Design review of the part built by this model. Coordinates are the model's own, in mm. A direction names the side the tool comes from. Coordinates: 2 decimals unless noted, no trailing zeros. Write each loop counter-clockwise with the first axis right and the second up, starting at its lowest first coordinate (ties: lowest second). Pieces come first, ordered by that corner, then holes. Notation, with made-up numbers: (35.25, 45.25) - (61.25, 45.25) arc R17 cw to (61.25, 69.25) - close; hole circle Ø9 at (71.5, 51). An arc over 180 degrees is marked (long way). Answer as a JSON object with one key per item and string values.
```python
from build123d import *

# Parameters (mm, degrees)
SKETCH1_W               = 5
SKETCH1_H               = 5
SKETCH1_R               = 0.95
CENTER_DEPTH            = 1.3
RIGHTSIDE_START         = 1.3
SKETCH1_2_W             = 5
SKETCH1_2_H             = 5
SKETCH1_2_R             = 0.95
RIGHTSIDE_DEPTH         = 1.2
LEFTSIDE_START          = -1.3
SKETCH1_3_W             = 5
SKETCH1_3_H             = 5
SKETCH1_3_R             = 0.95
LEFTSIDE_DEPTH          = 1.2
SKETCH3_W               = 5
SKETCH3_H               = 5
BOSS_EXTRUDE4_DEPTH     = 47.5
CUT_EXTRUDE1_DEPTH      = 5
CIRPATTERN2_COUNT       = 6
CIRPATTERN3_COUNT       = 3
CIRPATTERN4_START       = -44.601270189
CIRPATTERN4_OUTLINE_W   = 5
CIRPATTERN4_OUTLINE_H   = 5
CIRPATTERN4_OUTLINE_R   = 0.95
CIRPATTERN4_DEPTH       = 2.6
CIRPATTERN4_2_OUTLINE_W = 5
CIRPATTERN4_2_OUTLINE_H = 5
CIRPATTERN4_2_OUTLINE_R = 0.95
CIRPATTERN4_2_DEPTH     = 2.6
CIRPATTERN4_START_2     = -1.3
CIRPATTERN4_3_OUTLINE_W = 5
CIRPATTERN4_3_OUTLINE_H = 5
CIRPATTERN4_3_OUTLINE_R = 0.95
CIRPATTERN4_3_DEPTH     = 2.6
SKETCH5_W               = 5
SKETCH5_H               = 2.6
CUT_EXTRUDE2_DEPTH      = 5
INTERSECT1_START        = -46.716333699
INTERSECT1_OUTLINE_W    = 105
INTERSECT1_OUTLINE_H    = 5
INTERSECT1_OUTLINE_R    = 0.95
INTERSECT1_DEPTH        = 49.216333699


# Read off the part's stored shape, not the designer's step: CirPattern4, Intersect1
with BuildPart() as part:
    # Sketch1 → Center (new, symmetric)
    with BuildSketch(Plane(origin=(0, 0, 0), x_dir=(1, 0, 0), z_dir=(0, 1, 0))):
        Rectangle(SKETCH1_W, SKETCH1_H)
        with Locations(Location((0, 0, 0), (0, 0, 270))):
            Circle(SKETCH1_R, mode=Mode.SUBTRACT)
    extrude(amount=CENTER_DEPTH, both=True)

    # Sketch5 → Cut-Extrude2 (cut)
    with BuildSketch(Plane(origin=(2.5, 0, 0), x_dir=(0, 0, -1), z_dir=(1, 0, 0))):
        Rectangle(SKETCH5_W, SKETCH5_H)
    extrude(amount=-CUT_EXTRUDE2_DEPTH, mode=Mode.SUBTRACT)


with BuildPart() as body_2:
    # Sketch1<2> → RightSide (new body)
    with BuildSketch(Plane(origin=(0, 0, 0), x_dir=(1, 0, 0), z_dir=(0, 1, 0)).offset(RIGHTSIDE_START)):
        Rectangle(SKETCH1_2_W, SKETCH1_2_H)
        with Locations(Location((0, 0, 0), (0, 0, 270))):
            Circle(SKETCH1_2_R, mode=Mode.SUBTRACT)
    extrude(amount=RIGHTSIDE_DEPTH)


with BuildPart() as body_3:
    # Sketch1<3> → LeftSide (new body)
    with BuildSketch(Plane(origin=(0, 0, 0), x_dir=(1, 0, 0), z_dir=(0, 1, 0)).offset(LEFTSIDE_START)):
        Rectangle(SKETCH1_3_W, SKETCH1_3_H)
        with Locations(Location((0, 0, 0), (0, 0, 270))):
            Circle(SKETCH1_3_R, mode=Mode.SUBTRACT)
    extrude(amount=-LEFTSIDE_DEPTH)


with BuildPart() as body_4:
    # Sketch3 → Boss-Extrude4 (new body)
    with BuildSketch(Plane.ZY.offset(2.5)):
        Rectangle(SKETCH3_W, SKETCH3_H)
    extrude(amount=BOSS_EXTRUDE4_DEPTH)

    # Sketch4 → Cut-Extrude1 (cut)
    with BuildSketch(Plane.XY.offset(-2.5)):
        Polygon((-50, 0), (-50, -2.5), (-45.669872981, -2.5), align=None)
        Polygon((-50, 2.5), (-50, 0), (-45.669872981, 2.5), align=None)
    extrude(amount=CUT_EXTRUDE1_DEPTH, mode=Mode.SUBTRACT)


with BuildPart() as cirpattern2_1:
    # CirPattern2: pattern copy
    add(body_4.part.rotate(Axis((-50, 0, 0), (0, 0, 1)), 1 * 360 / CIRPATTERN2_COUNT))


with BuildPart() as cirpattern2_2:
    # CirPattern2: pattern copy
    add(body_4.part.rotate(Axis((-50, 0, 0), (0, 0, 1)), 2 * 360 / CIRPATTERN2_COUNT))


with BuildPart() as cirpattern2_3:
    # CirPattern2: pattern copy
    add(body_4.part.rotate(Axis((-50, 0, 0), (0, 0, 1)), 3 * 360 / CIRPATTERN2_COUNT))


with BuildPart() as cirpattern2_4:
    # CirPattern2: pattern copy
    add(body_4.part.rotate(Axis((-50, 0, 0), (0, 0, 1)), 4 * 360 / CIRPATTERN2_COUNT))


with BuildPart() as cirpattern2_5:
    # CirPattern2: pattern copy
    add(body_4.part.rotate(Axis((-50, 0, 0), (0, 0, 1)), 5 * 360 / CIRPATTERN2_COUNT))


with BuildPart() as cirpattern3_1:
    # CirPattern3: pattern copy
    add(body_3.part.rotate(Axis((-50, 0, 0), (0, 0, 1)), 1 * 360 / CIRPATTERN3_COUNT))


with BuildPart() as cirpattern3_2:
    # CirPattern3: pattern copy
    add(body_3.part.rotate(Axis((-50, 0, 0), (0, 0, 1)), 2 * 360 / CIRPATTERN3_COUNT))


with BuildPart() as cirpattern3_3:
    # CirPattern3: pattern copy
    add(body_2.part.rotate(Axis((-50, 0, 0), (0, 0, 1)), 1 * 360 / CIRPATTERN3_COUNT))


with BuildPart() as cirpattern3_4:
    # CirPattern3: pattern copy
    add(body_2.part.rotate(Axis((-50, 0, 0), (0, 0, 1)), 2 * 360 / CIRPATTERN3_COUNT))


with BuildPart() as body_14:
    # CirPattern4 outline → CirPattern4 (new body)
    with BuildSketch(Plane(origin=(0, 0, 0), x_dir=(0.49999999999999767, 0.86602540378444, 0), z_dir=(0.8660254037844399, -0.49999999999999795, 0)).offset(CIRPATTERN4_START)):
        with Locations((25, 0)):
            Rectangle(CIRPATTERN4_OUTLINE_W, CIRPATTERN4_OUTLINE_H)
        with Locations((25, 0)):
            Circle(CIRPATTERN4_OUTLINE_R, mode=Mode.SUBTRACT)
    extrude(amount=CIRPATTERN4_DEPTH)


with BuildPart() as body_15:
    # CirPattern4 2 outline → CirPattern4 2 (new body)
    with BuildSketch(Plane(origin=(0, 0, 0), x_dir=(0.5000000000000098, -0.8660254037844329, 0), z_dir=(0.8660254037844329, 0.50000000000001, 0)).offset(CIRPATTERN4_START)):
        with Locations((25, 0)):
            Rectangle(CIRPATTERN4_2_OUTLINE_W, CIRPATTERN4_2_OUTLINE_H)
        with Locations((25, 0)):
            Circle(CIRPATTERN4_2_OUTLINE_R, mode=Mode.SUBTRACT)
    extrude(amount=CIRPATTERN4_2_DEPTH)


with BuildPart() as body_16:
    # CirPattern4 3 outline → CirPattern4 3 (new body)
    with BuildSketch(Plane(origin=(0, 0, 0), x_dir=(1, 0, 0), z_dir=(0, 1, 0)).offset(CIRPATTERN4_START_2)):
        with Locations((-100, 0)):
            Rectangle(CIRPATTERN4_3_OUTLINE_W, CIRPATTERN4_3_OUTLINE_H)
        with Locations((-100, 0)):
            Circle(CIRPATTERN4_3_OUTLINE_R, mode=Mode.SUBTRACT)
    extrude(amount=CIRPATTERN4_3_DEPTH)


with BuildPart() as cirpattern2_5_1:
    add(cirpattern2_5.part)

    # Combine1: union CirPattern2_3, CirPattern2_4, body 16, CirPattern3_2, CirPattern3_4, body 15, CirPattern2_1, body 3, body 14, body 4, body 2, CirPattern2_2, CirPattern3_1, CirPattern3_3
    add(cirpattern2_3.part)
    add(cirpattern2_4.part)
    add(body_16.part)
    add(cirpattern3_2.part)
    add(cirpattern3_4.part)
    add(body_15.part)
    add(cirpattern2_1.part)
    add(body_3.part)
    add(body_14.part)
    add(body_4.part)
    add(body_2.part)
    add(cirpattern2_2.part)
    add(cirpattern3_1.part)
    add(cirpattern3_3.part)

    # Intersect1 outline → Intersect1 (cut)
    with BuildSketch(Plane(origin=(0, 0, 0), x_dir=(1, 0, 0), z_dir=(0, 1, 0)).offset(INTERSECT1_START)):
        with Locations((-50, 0)):
            Rectangle(INTERSECT1_OUTLINE_W, INTERSECT1_OUTLINE_H)
        with Locations((-100, 0)):
            Circle(INTERSECT1_OUTLINE_R, mode=Mode.SUBTRACT)
        Circle(INTERSECT1_OUTLINE_R, mode=Mode.SUBTRACT)
    extrude(amount=INTERSECT1_DEPTH, mode=Mode.SUBTRACT)


solid = cirpattern2_5_1.part
```
(1) Take a section at D-D, the plane x = -53.5. Write out the cut boundary in (y, z), and give its area (3 significant figures).
Solved:
{"outline": "(2.5, -2.5) - (11.06, -2.5) - (11.06, 2.5) - (2.5, 2.5) - close", "area": "42.8 mm^2"}
(2) Tool access review of faces 1 (the face through (-23.89, 42.62, 1.15)), 2 (the face through (-73.766, 41.127, -0.035)), 3 (the face through (-58.3, 18.6, 2.5)), 4 (the face through (-39.06, 23.95, -0.03)), 5 (the face through (-25.49, 42.49, 0.04)): name each direction out of +Z, -Z, +X, -X, +Y, -Y from which nothing blocks a thin tool from reaching the whole face with its end or side.
Solved:
{"face 1": "+Z, -Z, +X", "face 2": "+Z, -Z", "face 3": "+Z, +X, -X, +Y, -Y", "face 4": "+Z, -Z, +Y", "face 5": "none"}
(3) Take a section at B-B, the plane z = -1.55. Write out the cut boundary in (x, y), and give its area (3 significant figures).
Solved:
{"outline": "(-78.42, 44.22) - (-54.33, 2.5) - (-45.67, 2.5) - (-24.08, 39.89) - (-25.12, 40.49) - (-22.62, 44.82) - (-24.88, 46.12) - (-27.38, 41.79) - (-28.42, 42.39) - (-50, 5) - (-74.08, 46.72) - (-75.12, 46.12) - (-72.62, 41.79) - (-74.88, 40.49) - (-77.38, 44.82) - close", "area": "468 mm^2"}
(4) For pin 1 (3 mm diameter, centred on y = 20, z = 1, fed in from -X); pin 2 (1 mm diameter, centred on y = 12, z = 0, fed in from -X); pin 3 (2 mm diameter, centred on x = -30, z = 0.5, fed in from -Y), all flat-tipped, find the tip position at first contact; note any pin that passes through.
Solved:
{"pin 1": "stops at x = -65.3", "pin 2": "stops at x = -60.1", "pin 3": "stops at y = 27.91"}
(5) To check wall thickness, follow line 1 (X direction, y = 17, z = -1.3); line 2 (X direction, y = 32.5, z = -0.4); line 3 (Y direction, x = -28.5, z = -0.1). State the ranges of each line that lie inside material, in increasing order. Write a range as from..to.
Solved:
{"line 1": "x = -62.7..-56.93, -43.07..-37.3", "line 2": "x = -71.65..-65.88, -34.12..-28.35", "line 3": "y = 32.24..42.24"}
(6) Take a section at A-A, the plane y = 6. Write out the cut boundary in (x, z), and give its area (3 significant figures).
Solved:
{"outline": "(-56.35, -2.5) - (-50.58, -2.5) - (-50.58, 2.5) - (-56.35, 2.5) - close; (-49.42, -2.5) - (-43.65, -2.5) - (-43.65, 2.5) - (-49.42, 2.5) - close", "area": "57.7 mm^2"}
(7) Take a section at C-C, the plane x = -32.5. Write out the cut boundary in (y, z), and give its area (3 significant figures).
Solved:
{"outline": "(25.31, -2.5) - (35.31, -2.5) - (35.31, 2.5) - (25.31, 2.5) - close", "area": "50.0 mm^2"}
(8) The part is to be moulded in two halves that separate along X. For faces 6 (the face through (-50, 2.5, 0)), 7 (the face through (-34.7, 21.5, 0)), 8 (the face through (-66.204, 23.066, -0.035)), 9 (the face through (-26.7, 42.96, 0.04)), say which applies: pulls with the +X half, pulls with the -X half, needs draft (parallel to the pull), parting line crosses it, or undercut.
Solved:
{"face 6": "needs draft", "face 7": "pulls with the +X half", "face 8": "pulls with the -X half", "face 9": "undercut"}
